Here's how the part is built. I have some questions about the finished solid (model axes, mm). A direction names the side the tool comes from. Give positions to 0.01 mm unless a question says otherwise; leave off trailing zeros. Write each loop counter-clockwise with the first axis right and the second up, starting at its lowest first coordinate (ties: lowest second). Pieces come first, ordered by that corner, then holes. Notation, with made-up numbers: (23, 10) -> (79, 10) arc R9 ccw to (79, 14) -> close; hole circle Ø5 at (83.5, 7). An arc over 180 degrees is marked (long way). Put each result on its own line as item: value. Start each with the question number.
from build123d import *

# Parameters (mm, degrees)
SKETCH1_W           = 140
SKETCH1_H           = 15
BOSS_EXTRUDE1_DEPTH = 30
SKETCH2_W           = 122
SKETCH2_H           = 27
CUT_EXTRUDE1_DEPTH  = 30
SKETCH3_W           = 13
SKETCH3_H           = 27
CUT_EXTRUDE2_DEPTH  = 144.689142732
BOSS_EXTRUDE2_REACH = 119.876
SKETCH4_W           = 2
SKETCH4_H           = 13
CUT_EXTRUDE3_DEPTH  = 144.689142732
SKETCH6_R           = 1.6
CUT_EXTRUDE4_DEPTH  = 118.971522149
SKETCH7_R           = 2.1
CUT_EXTRUDE5_DEPTH  = 30
SKETCH8_W           = 122
SKETCH8_H           = 2
BOSS_EXTRUDE3_DEPTH = 5
FILLET3_R           = 10
FILLET4_R           = 2


with BuildPart() as part:
    # Sketch1 → Boss-Extrude1 (new body)
    with BuildSketch(Plane(origin=(0, 0, 0), x_dir=(1, 0, 0), z_dir=(0, 1, 0))):
        with Locations((-43.350253807, -4.606598985)):
            Rectangle(SKETCH1_W, SKETCH1_H)
    extrude(amount=BOSS_EXTRUDE1_DEPTH)

    # Sketch2 → Cut-Extrude1 (cut)
    with BuildSketch(Plane.XY.offset(12.106598985)):
        with Locations((-43.350253807, 16.5)):
            Rectangle(SKETCH2_W, SKETCH2_H)
    extrude(amount=-CUT_EXTRUDE1_DEPTH, mode=Mode.SUBTRACT)

    # Sketch3 → Cut-Extrude2 (cut, through all)
    with BuildSketch(Plane.ZY.offset(113.350253807)):
        with Locations((3.606598985, 16.5)):
            Rectangle(SKETCH3_W, SKETCH3_H)
    extrude(amount=-CUT_EXTRUDE2_DEPTH, mode=Mode.SUBTRACT)

    # Sketch4 → Boss-Extrude2 (add, up to next)
    with BuildSketch(Plane(origin=(0, 30, 0), x_dir=(1, 0, 0), z_dir=(0, 1, 0)), mode=Mode.PRIVATE) as boss_extrude2_sk1:
        with Locations((25.649746193, -3.606598985)):
            Rectangle(SKETCH4_W, SKETCH4_H)
    boss_extrude2_tool1 = extrude(boss_extrude2_sk1.sketch, amount=-BOSS_EXTRUDE2_REACH, mode=Mode.PRIVATE) - part.part
    # Sketch4 → Boss-Extrude2 (add, up to next)
    with BuildSketch(Plane(origin=(0, 30, 0), x_dir=(1, 0, 0), z_dir=(0, 1, 0)), mode=Mode.PRIVATE) as boss_extrude2_sk2:
        with Locations((-112.350253807, -3.606598985)):
            Rectangle(SKETCH4_W, SKETCH4_H)
    boss_extrude2_tool2 = extrude(boss_extrude2_sk2.sketch, amount=-BOSS_EXTRUDE2_REACH, mode=Mode.PRIVATE) - part.part
    add(boss_extrude2_tool1.solids().sort_by_distance((25.649746, 30, 3.606599))[0])
    add(boss_extrude2_tool2.solids().sort_by_distance((-112.350254, 30, 3.606599))[0])

    # Sketch5 → Cut-Extrude3 (cut, through all)
    with BuildSketch(Plane.ZY.offset(113.350253807)):
        Polygon((10.106598985, 30), (-2.893401015, 3), (-2.893401015, 30), align=None)
    extrude(amount=-CUT_EXTRUDE3_DEPTH, mode=Mode.SUBTRACT)

    # Sketch6 → Cut-Extrude4 (cut, through all)
    with BuildSketch(Plane(origin=(0, 0, 10.106598985), x_dir=(-1, 0, 0), z_dir=(0, 0, -1))):
        with Locations((-20.649746193, 25)):
            Circle(SKETCH6_R)
        with Locations((-20.649746193, 15)):
            Circle(SKETCH6_R)
        with Locations((107.350253807, 25)):
            Circle(SKETCH6_R)
        with Locations((107.350253807, 15)):
            Circle(SKETCH6_R)
    extrude(amount=-CUT_EXTRUDE4_DEPTH, mode=Mode.SUBTRACT)

    # Sketch7 → Cut-Extrude5 (cut)
    with BuildSketch(Plane(origin=(0, 3, 0), x_dir=(1, 0, 0), z_dir=(0, 1, 0))):
        with Locations(Location((-3.500253807, -4.106598985, 0), (0, 0, 270))):
            Circle(SKETCH7_R)
        with Locations(Location((-83.200253807, -4.106598985, 0), (0, 0, 270))):
            Circle(SKETCH7_R)
    extrude(amount=-CUT_EXTRUDE5_DEPTH, mode=Mode.SUBTRACT)

    # Sketch8 → Boss-Extrude3 (add)
    with BuildSketch(Plane(origin=(0, 3, 0), x_dir=(1, 0, 0), z_dir=(0, 1, 0))):
        with Locations((-43.350253807, -11.106598985)):
            Rectangle(SKETCH8_W, SKETCH8_H)
    extrude(amount=BOSS_EXTRUDE3_DEPTH)

    # Fillet3
    fillet3_edges = [part.edges().sort_by_distance(p)[0] for p in [
        (17.649746193, 8, 11.106598985),
        (-104.350253807, 8, 11.106598985),
    ]]
    fillet(fillet3_edges, radius=FILLET3_R)

    # Fillet4
    fillet4_edges = [part.edges().sort_by_distance(p)[0] for p in [
        (-43.350253807, 3, 10.106598985),
    ]]
    fillet(fillet4_edges, radius=FILLET4_R)


solid = part.part
1) I'm going to push flat-ended pins straight in: pin 1 Ø1.6 at (x, z) = (-38, 11) entering from +Y; pin 2 Ø5 at (x, z) = (-70.5, 5) entering from +Y; pin 3 Ø4 at (x, z) = (-3.5, 4.11) entering from -Y; pin 4 Ø4 at (x, y) = (-107.35, 15) entering from -Z. Where does each tip first touch, or does it pass through?
2) I need wall thicknesses on probe 1 along Y at (x, z) = (-80.5, 7.75); probe 2 along Z at (x, y) = (-0.5, 7.25); probe 3 along X at (y, z) = (18.75, 7.5). Which ranges of each line are inside material? Lowest first, please.
3) I want a section at C-C, the plane y = 25. Write out the boundary of the cut face in (x, z).
4) I want a section at A-A, the plane y = 15. Write out the boundary of the cut face in (x, z).
5) I want a section at B-B, the plane x = -35. Write out the boundary of the cut face in (y, z).
6) I want a section at D-D, the plane x = 14. Write out the boundary of the cut face in (y, z).
7) Which directions (+Z, -Z, +X, -X, +Y, -Y) give clear straight access to the entire face, cutting with the end or side of a thin tool? Please do faces 5 (the cylindrical face through (-85.25, 1.52, 3.65)), 6 (the flat face through (-49, 7, 10.107)), 7 (the cylindrical face through (-101.5, 11.01, 11.09)).
8) Thinking about a two-plate mould opening in Y: for faces 1 (the cylindrical face through (-108.876, 25.481, 11.093)), 2 (the flat face through (24.65, 11, 7)), 3 (the cylindrical face through (-108.876, 15.481, 11.093)), 4 (the cylindrical face through (14.8, 11.01, 11.09)), which applies, released by +Y, released by -Y, zero draft, split by the parting line, or undercut?
Established:
1. pin 1: stops at y = 8
1. pin 2: stops at y = 3
1. pin 3: passes through
1. pin 4: stops at z = 10.11
2. probe 1: y = 0 to 3
2. probe 2: z = 10.11 to 12.11
2. probe 3: x = -113.35 to -111.35, 24.65 to 26.65
3. outline: (-113.35, 7.7) -> (-111.35, 7.7) -> (-111.35, 10.11) -> (-108.95, 10.11) -> (-108.95, 12.11) -> (-113.35, 12.11) -> close; (-105.75, 10.11) -> (-104.35, 10.11) -> (-104.35, 12.11) -> (-105.75, 12.11) -> close; (17.65, 10.11) -> (19.05, 10.11) -> (19.05, 12.11) -> (17.65, 12.11) -> close; (22.25, 10.11) -> (24.65, 10.11) -> (24.65, 7.7) -> (26.65, 7.7) -> (26.65, 12.11) -> (22.25, 12.11) -> close
4. outline: (-113.35, 2.88) -> (-111.35, 2.88) -> (-111.35, 10.11) -> (-108.95, 10.11) -> (-108.95, 12.11) -> (-113.35, 12.11) -> close; (-105.75, 10.11) -> (-103.89, 10.11) -> (-103.89, 12.11) -> (-105.75, 12.11) -> close; (17.19, 10.11) -> (19.05, 10.11) -> (19.05, 12.11) -> (17.19, 12.11) -> close; (22.25, 10.11) -> (24.65, 10.11) -> (24.65, 2.88) -> (26.65, 2.88) -> (26.65, 12.11) -> (22.25, 12.11) -> close
5. outline: (0, -2.89) -> (3, -2.89) -> (3, 8.11) arc R2 cw to (5, 10.11) -> (8, 10.11) -> (8, 12.11) -> (0, 12.11) -> close
6. outline: (0, -2.89) -> (3, -2.89) -> (3, 8.11) arc R2 cw to (5, 10.11) -> (10.28, 10.11) -> (10.28, 12.11) -> (0, 12.11) -> close
7. face 5: +Y, -Y
7. face 6: -Z, +Y
7. face 7: +Z, -Z, +Y
8. face 1: undercut
8. face 2: zero draft
8. face 3: undercut
8. face 4: released by +Y
